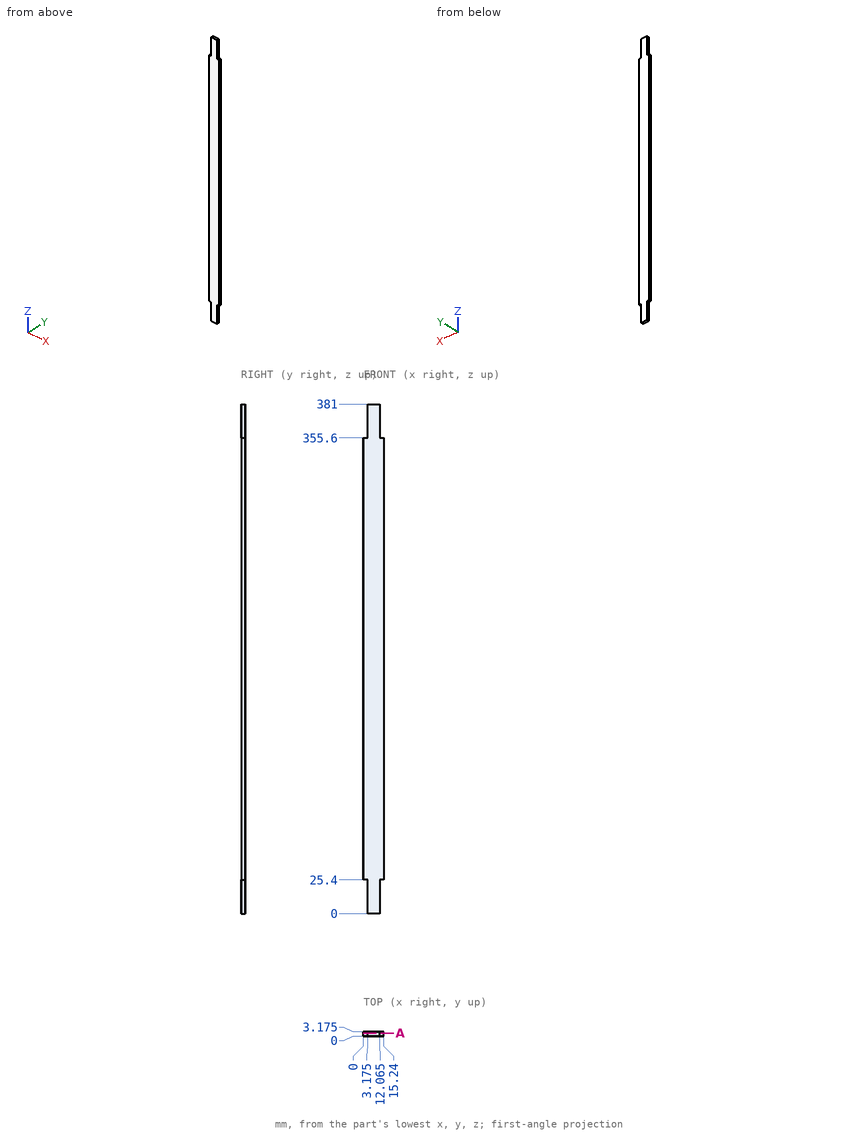
Part print with two shaded views. Sizes in mm from the minimum x, y, z corner. Coordinates: 2 decimals unless noted, no trailing zeros. Order: outer loops, then holes, each group sorted by start corner. A loop starts at its lowest first (then second) coordinate and runs counter-clockwise, first axis right, second up.
(1) Saw through at A-A, the plane y = 2.15. Write the cut outline in (x, z) (3 decimals), and give its area (3 significant figures).
Solution:
outline: (0, 25.4) - (3.175, 25.4) - (3.175, 0) - (12.065, 0) - (12.065, 25.4) - (15.24, 25.4) - (15.24, 355.6) - (12.065, 355.6) - (12.065, 381) - (3.175, 381) - (3.175, 355.6) - (0, 355.6) - close
area: 5,480 mm2
(2) Pin check, flat tips, straight feed: pin 1 Ø1 at (x, y) = (13, 1.5) entering from -Z; pin 2 Ø1 at (y, z) = (1.5, 16.5) entering from +X (3 decimals); pin 3 Ø1.6 at (y, z) = (1.5, 16.5) entering from -X (3 decimals). Stop position of each tip, or through.
Solution:
pin 1: stops at z = 25.4
pin 2: stops at x = 12.065
pin 3: stops at x = 3.175
(3) Drill centre lines: L1, parallel to X at y = 0.75, z = 15.5 (3 decimals); L2, parallel to Z at x = 14.75, y = 1.7. Where is each one in solid material? Low to high.
Solution:
L1: x = 3.175 to 12.065
L2: z = 25.4 to 355.6
